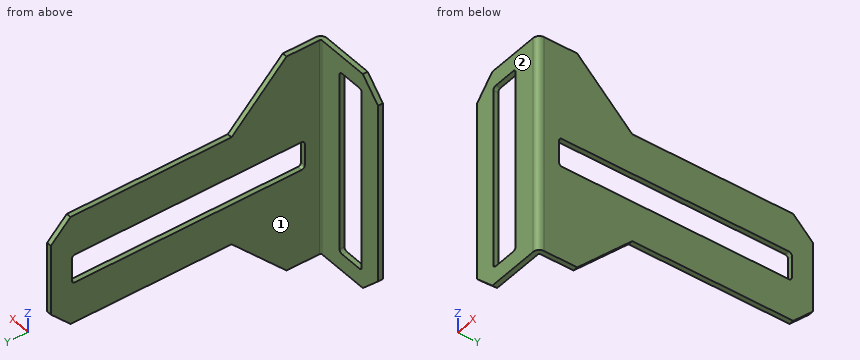
```python
from build123d import *

# Parameters (mm, degrees)
SKETCH1_W           = 44.45
SKETCH1_H           = 35.56
BOSS_EXTRUDE1_DEPTH = 12.7
SKETCH2_W           = 11.9126
SKETCH2_H           = 43.6626
CUT_EXTRUDE1_DEPTH  = 36.56
SKETCH3_W           = 8.89
SKETCH3_H           = 29.21
CUT_EXTRUDE2_DEPTH  = 13.7
SKETCH4_W           = 8.89
SKETCH4_H           = 38.1
CUT_EXTRUDE3_DEPTH  = 13.7
SKETCH5_W           = 4.6228
SKETCH5_H           = 30.0228
CUT_EXTRUDE4_DEPTH  = 45.45
SKETCH6_W           = 4.6228
SKETCH6_H           = 37.6428
CUT_EXTRUDE5_DEPTH  = 13.7
DRAFT1_ANGLE        = 45
DRAFT2_ANGLE        = 45
CHAMFER1_SIZE       = 3.175
FILLET1_R           = 0.2032
FILLET2_R           = 0.508
FILLET3_R           = 0.9906


with BuildPart() as part:
    # Sketch1 → Boss-Extrude1 (new body)
    with BuildSketch(Plane(origin=(0, 0, 0), x_dir=(0, -1, 0), z_dir=(-1, 0, 0))):
        with Locations((-22.225, 0)):
            Rectangle(SKETCH1_W, SKETCH1_H)
    extrude(amount=-BOSS_EXTRUDE1_DEPTH)

    # Sketch2 → Cut-Extrude1 (cut, through all)
    with BuildSketch(Plane(origin=(0, 0, -17.78), x_dir=(-1, 0, 0), z_dir=(0, 0, -1))):
        with Locations((-5.9563, 22.6187)):
            Rectangle(SKETCH2_W, SKETCH2_H)
    extrude(amount=-CUT_EXTRUDE1_DEPTH, mode=Mode.SUBTRACT)

    # Sketch3 → Cut-Extrude2 (cut, through all)
    with BuildSketch(Plane(origin=(12.7, 0, 0), x_dir=(0, 0, -1), z_dir=(1, 0, 0))):
        with Locations((13.335, 29.845)):
            Rectangle(SKETCH3_W, SKETCH3_H)
    extrude(amount=-CUT_EXTRUDE2_DEPTH, mode=Mode.SUBTRACT)

    # Sketch4 → Cut-Extrude3 (cut, through all)
    with BuildSketch(Plane(origin=(12.7, 0, 0), x_dir=(0, 0, -1), z_dir=(1, 0, 0))):
        with Locations((-13.335, 25.4)):
            Rectangle(SKETCH4_W, SKETCH4_H)
    extrude(amount=-CUT_EXTRUDE3_DEPTH, mode=Mode.SUBTRACT)

    # Sketch5 → Cut-Extrude4 (cut, through all)
    with BuildSketch(Plane.XZ):
        with Locations((5.715, 0)):
            Rectangle(SKETCH5_W, SKETCH5_H)
    extrude(amount=-CUT_EXTRUDE4_DEPTH, mode=Mode.SUBTRACT)

    # Sketch6 → Cut-Extrude5 (cut, through all)
    with BuildSketch(Plane(origin=(12.7, 0, 0), x_dir=(0, 0, -1), z_dir=(1, 0, 0))):
        with Locations((0, 22.225)):
            Rectangle(SKETCH6_W, SKETCH6_H)
    extrude(amount=-CUT_EXTRUDE5_DEPTH, mode=Mode.SUBTRACT)

    # Draft1
    draft1_faces = [part.faces().sort_by_distance(p)[0] for p in [
        (12.3063, 15.24, -13.335),
    ]]
    draft(draft1_faces, Plane(origin=(0, 44.45, -8.89), x_dir=(-1, 0, 0), z_dir=(0, 0, -1)), DRAFT1_ANGLE)

    # Draft2
    draft2_faces = [part.faces().sort_by_distance(p)[0] for p in [
        (12.3063, 6.35, 13.335),
    ]]
    draft(draft2_faces, Plane(origin=(12.7, 0, 17.78), x_dir=(1, 0, 0), z_dir=(0, 0, 1)), DRAFT2_ANGLE)

    # Chamfer1
    chamfer1_edges = [part.edges().sort_by_distance(p)[0] for p in [
        (0, 0.3937, -17.78),
        (12.3063, 44.45, -8.89),
        (0, 0.3937, 17.78),
        (12.3063, 44.45, 8.89),
    ]]
    chamfer(chamfer1_edges, length=CHAMFER1_SIZE)

    # Fillet1
    fillet1_edges = [part.edges().sort_by_distance(p)[0] for p in [
        (11.9126, 0.7874, 0),
    ]]
    fillet(fillet1_edges, radius=FILLET1_R)

    # Fillet2
    fillet2_edges = [part.edges().sort_by_distance(p)[0] for p in [
        (8.0264, 0.3937, 15.0114),
        (8.0264, 0.3937, -15.0114),
        (3.4036, 0.3937, -15.0114),
        (3.4036, 0.3937, 15.0114),
        (12.3063, 41.0464, 2.3114),
        (12.3063, 41.0464, -2.3114),
        (12.3063, 3.4036, -2.3114),
        (12.3063, 3.4036, 2.3114),
    ]]
    fillet(fillet2_edges, radius=FILLET2_R)

    # Fillet3
    fillet3_edges = [part.edges().sort_by_distance(p)[0] for p in [
        (12.7, 0, 0),
    ]]
    fillet(fillet3_edges, radius=FILLET3_R)


solid = part.part
```
For this review, take the finished solid that the model builds, in its own axes (mm). Face numbers are marked on the shaded views. A direction names the side the tool comes from. Round coordinates to 2 decimals unless told otherwise and drop trailing zeros. Write each loop counter-clockwise with the first axis right and the second up, starting at its lowest first coordinate (ties: lowest second). Pieces come first, ordered by that corner, then holes. Notation, with made-up numbers: (16.5, 88) - (27.5, 88) arc R28 cw to (27.5, 114) - close; hole circle Ø11 at (49, 79). An arc over 180 degrees is marked (long way). Put each result on its own line as item: value.
Q1. Machinability: for the marked faces 1 and 2, which of the approach directions +Z, -Z, +X, -X, +Y, -Y give a long, thin tool a straight path to every point of the face, cutting with its end or side? Answer none if there is none.
Solved:
face 1: +Z, -Z, -X, +Y
face 2: +Z, -Z, +X, -X, -Y
Q2. We need section C-C (z = 3). Give the boundary of the cut face in (x, y), and give its area (3 significant figures).
Solved:
outline: (0, 0) - (3.4, 0) - (3.4, 0.79) - (0, 0.79) - close; (8.03, 0) - (11.71, 0) arc R0.99 ccw to (12.7, 0.99) - (12.7, 44.45) - (11.91, 44.45) - (11.91, 0.99) arc R0.2 cw to (11.71, 0.79) - (8.03, 0.79) - close
area: 40.5 mm2
Q3. We need section D-D (z = -9.5). Give the boundary of the cut face in (x, y), and give its area (3 significant figures).
Solved:
outline: (0, 0) - (3.4, 0) - (3.4, 0.79) - (0, 0.79) - close; (8.03, 0) - (11.71, 0) arc R0.99 ccw to (12.7, 0.99) - (12.7, 14.63) - (11.91, 14.63) - (11.91, 0.99) arc R0.2 cw to (11.71, 0.79) - (8.03, 0.79) - close
area: 17.1 mm2
Q4. We need section B-B (y = 39.5). Give the boundary of the cut face in (x, z), and give its area (3 significant figures).
Solved:
outline: (11.91, -8.89) - (12.7, -8.89) - (12.7, -2.31) - (11.91, -2.31) - close; (11.91, 2.31) - (12.7, 2.31) - (12.7, 8.89) - (11.91, 8.89) - close
area: 10.4 mm2
Q5. We need section A-A (x = 4.75). Give the boundary of the cut face in (y, z).
Solved:
outline: (0, -17.78) - (0.79, -17.78) - (0.79, -15.01) - (0, -15.01) - close; (0, 15.01) - (0.79, 15.01) - (0.79, 17.78) - (0, 17.78) - close
Q6. Wall thickness on probe 1 along Y at (x, z) = (9.5, 11); probe 2 along X at (y, z) = (16, 6.5); probe 3 along Y at (x, z) = (12, -10): over which ranges is each line inside the solid? List them lowest first.
Solved:
probe 1: y = 0 to 0.79
probe 2: x = 11.91 to 12.7
probe 3: y = 0.04 to 14.13
Q7. Insertion check: pin 1 Ø0.6 at (x, y) = (12.5, 26.5) entering from -Z; pin 2 Ø0.9 at (x, y) = (12.5, 30.5) entering from +Z; pin 3 Ø18 at (y, z) = (27.5, -8) entering from -X; pin 4 Ø6 at (x, z) = (4.5, 1.5) entering from -Y. Each pin has a flat end and moves straight along its axis. Give the tip position at first contact, or say it passes through.
Solved:
pin 1: stops at z = -8.89
pin 2: stops at z = 8.89
pin 3: stops at x = 11.91
pin 4: stops at y = 0
